Source: CAD feature listing. Evaluate the final solid. Frame: model axes, mm. A direction names the side the tool comes from. Coordinates: 2 decimals unless noted, no trailing zeros. Loops run counter-clockwise (first coordinate to the right, second up) from the corner with the lowest first, then second, coordinate; pieces in that order, holes last. Notation, with made-up numbers: (-37.75, 72) -> (-20.75, 72) arc R19 cw to (-20.75, 79) -> close; hole circle Ø10 at (37, -29.5). An arc over 180 degrees is marked (long way). Answer as CSV lines item,"result".
Autodesk Inventor part; units mm, degrees
ref_plane "РабПлоскость1" through (14, 8, 0) normal (0, 1, 0) x (-1, 0, 0)
ref_plane "YZ Plane" through (0, 0, 0) normal (1, 0, 0) x (0, 1, 0)
ref_plane "XY Plane" through (0, 0, 0) normal (0, 0, 1) x (1, 0, 0)
sketch "Эскиз1" plane through (0, 0, 0) normal (0, 0, 1) x (1, 0, 0)
  line L0 (10, 6.11) -> (10, 8)
  line L1 (10, 8) -> (18, 8)
  line L2 (18, 8) -> (18, 6.11)
  line L3 (18, 6.11) -> (27, 6.11)
  line L4 (27, 6.11) -> (27, 8)
  line L5 (27, 8) -> (28, 8)
  line L6 (28, 8) -> (28, 0)
  line L7 (0, 0) -> (0, 8)
  line L8 (0, 8) -> (1, 8)
  line L9 (1, 8) -> (1, 6.11)
  line L10 (1, 6.11) -> (10, 6.11)
  line L11 (0, 0) -> (28, 0)
  point P0 (22.5, 6.11)
  dimension "d0" = 6.11
  dimension "d1" = 8
  dimension "d2" = 28
  dimension "d4" = 9
  dimension "d5" = 8
revolve "Вращение1" add sketch "Эскиз1" angle 360 about axis through (0, 0, 0) along (1, 0, 0)
sketch "Эскиз2" plane through (28, 0, 0) normal (1, 0, 0) x (0, 0, -1)
  circle A0 centre (0, 0) radius 4
  dimension "d7" = 8
extrude "Выдавливание1" cut sketch "Эскиз2" against normal through all
ref_plane "РабПлоскость1" through (14, 8, 0) normal (0, 1, 0) x (-1, 0, 0)
sketch "Эскиз3" plane through (14, 8, 0) normal (0, 1, 0) x (-1, 0, 0)
  circle A0 centre (0, 0) radius 2
  line L0 (4, -8) -> (-4, -8)
  point P0 (14, 0)
  point P1 (0, -8)
  dimension "d10" = 4
extrude "Выдавливание2" cut sketch "Эскиз3" against normal blind 6.5
pattern_circular "Круговой массив1" count 2 over 90 about axis through (14, 0, 0) along (1, 0, 0) of "Выдавливание2"
properties part number "double_gt2"
(1) Material intervals for L1, parallel to X at y = 2, z = -6; L2, parallel to X at y = 6.45, z = 0; L3, parallel to X at y = 0, z = 6.05, sorted ascending. Write a range as [from, to].
Computed values:
L1,"[0, 1], [10, 18], [27, 28]"
L2,"[0, 1], [10, 12], [16, 18], [27, 28]"
L3,"[0, 12], [16, 28]"
(2) Cut plane C-C (z = 0). Return the cut outline in (x, y), then the cut area to 3 significant figures.
Computed values:
outline,"(0, -8) -> (1, -8) -> (1, -6.11) -> (10, -6.11) -> (10, -8) -> (18, -8) -> (18, -6.11) -> (27, -6.11) -> (27, -8) -> (28, -8) -> (28, -4) -> (0, -4) -> close; (0, 4) -> (12, 4) -> (12, 8) -> (10, 8) -> (10, 6.11) -> (1, 6.11) -> (1, 8) -> (0, 8) -> close; (16, 4) -> (28, 4) -> (28, 8) -> (27, 8) -> (27, 6.11) -> (18, 6.11) -> (18, 8) -> (16, 8) -> close"
area,"140 mm^2"
(3) Access query for faces 1 (the cylindrical face through (12.092, -0.601, 5.764)), 2 (the cylindrical face through (12.092, 5.764, 0.601)), 3 (the flat face through (10, -2, -6)). Directions: +Z, -Z, +X, -X, +Y, -Y. A direction counts if a zero-diameter tool reaches every point of the face in a straight line with its end or side. Return the directions, or none.
Computed values:
face 1,"+Z"
face 2,"+Y"
face 3,"none"
(4) Cut plane B-B (y = 6.75). Return the cut outline in (x, z), then the cut area to 3 significant figures.
Computed values:
outline,"(0, -4.29) -> (1, -4.29) -> (1, 4.29) -> (0, 4.29) -> close; (10, -4.29) -> (18, -4.29) -> (18, 4.29) -> (10, 4.29) -> close; (27, -4.29) -> (28, -4.29) -> (28, 4.29) -> (27, 4.29) -> close; hole circle Ø4 at (14, 0)"
area,"73.3 mm^2"
(5) Cut plane A-A (z = 6.5). Return the cut outline in (x, y), then the cut area to 3 significant figures.
Computed values:
outline,"(0, -4.66) -> (1, -4.66) -> (1, 4.66) -> (0, 4.66) -> close; (10, -4.66) -> (18, -4.66) -> (18, 4.66) -> (10, 4.66) -> close; (27, -4.66) -> (28, -4.66) -> (28, 4.66) -> (27, 4.66) -> close; hole circle Ø4 at (14, 0)"
area,"80.7 mm^2"
(6) Pin query (flat end, axial travel): pin 1 Ø2 at (x, z) = (4.5, 4) entering from +Y; pin 2 Ø1.5 at (x, z) = (20.5, 1.5) entering from +Y; pin 3 Ø3 at (x, y) = (14, -3.5) entering from -Z. Return the tip coordinate at first contact, or that it passes through.
Computed values:
pin 1,"y = 5.32"
pin 2,"y = 6.06"
pin 3,"z = -7.75"
(7) Draft query along Y for faces 4 (the cylindrical face through (14.196, -3.549, -1.846)), 5 (the flat face through (28, -4, -2)), 6 (the cylindrical face through (5.563, 5.828, 1.835)). Return one class per face: released by +Y, released by -Y, zero draft, split by the parting line, or undercut.
Computed values:
face 4,"undercut"
face 5,"zero draft"
face 6,"split by the parting line"
